from build123d import *

# Parameters (mm, degrees)
SKETCH_1_W           = 72
SKETCH_1_H           = 100
EXTRUDE_1_DEPTH      = 12
SKETCH_2_R           = 1.5
CUT_EXTRUDE_1_DEPTH  = 13
SKETCH_4_R           = 1.5
CUT_EXTRUDE_3_DEPTH  = 15
SKETCH_5_R           = 14.5
EXTRUDE_2_DEPTH      = 3.8
SKETCH_6_R           = 1.9
CUT_EXTRUDE_6_DEPTH  = 20
SKETCH_7_R           = 3.65
CUT_EXTRUDE_7_DEPTH  = 4.2
SKETCH_8_R           = 2.9
CUT_EXTRUDE_8_DEPTH  = 3.2
SKETCH_9_W           = 72
SKETCH_9_H           = 26
CUT_EXTRUDE_9_DEPTH  = 5.6
FILLET_1_R           = 5
SKETCH_10_W          = 10
SKETCH_10_H          = 100
CUT_EXTRUDE_10_DEPTH = 20
SKETCH_11_W          = 12
SKETCH_11_H          = 48
EXTRUDE_3_DEPTH      = 11
SKETCH_12_R          = 1.5
CUT_EXTRUDE_11_DEPTH = 50
SKETCH_14_W          = 12
SKETCH_14_H          = 25
CUT_EXTRUDE_12_DEPTH = 11
FILLET_2_R           = 6
FILLET_3_R           = 5


with BuildPart() as part:
    # 草图1 → 凸台-拉伸1 (new body)
    with BuildSketch(Plane.XY):
        Rectangle(SKETCH_1_W, SKETCH_1_H)
    extrude(amount=EXTRUDE_1_DEPTH)

    # 草图2 → 切除-拉伸1 (cut)
    with BuildSketch(Plane(origin=(0, 0, 0), x_dir=(-1, 0, 0), z_dir=(0, 0, -1))):
        with Locations((-28, 16)):
            Circle(SKETCH_2_R)
        with Locations((-28, -16)):
            Circle(SKETCH_2_R)
    extrude(amount=-CUT_EXTRUDE_1_DEPTH, mode=Mode.SUBTRACT)

    # 草图4 → 切除-拉伸3 (cut)
    with BuildSketch(Plane(origin=(0, 0, 0), x_dir=(-1, 0, 0), z_dir=(0, 0, -1))):
        with Locations((-32, 46)):
            Circle(SKETCH_4_R)
        with Locations((22, 46)):
            Circle(SKETCH_4_R)
        with Locations((-32, -46)):
            Circle(SKETCH_4_R)
        with Locations((22, -46)):
            Circle(SKETCH_4_R)
    extrude(amount=-CUT_EXTRUDE_3_DEPTH, mode=Mode.SUBTRACT)

    # 草图5 → 凸台-拉伸2 (add)
    with BuildSketch(Plane(origin=(0, 0, 0), x_dir=(-1, 0, 0), z_dir=(0, 0, -1))):
        with Locations(Location((0, 0, 0), (0, 0, 180))):
            Circle(SKETCH_5_R)
    extrude(amount=EXTRUDE_2_DEPTH)

    # 草图6 → 切除-拉伸6 (cut)
    with BuildSketch(Plane(origin=(0, 0, -3.8), x_dir=(-1, 0, 0), z_dir=(0, 0, -1))):
        with Locations((0, 11)):
            Circle(SKETCH_6_R)
        with Locations((9.526279442, 5.5)):
            Circle(SKETCH_6_R)
        with Locations((9.526279442, -5.5)):
            Circle(SKETCH_6_R)
        with Locations((0, -11)):
            Circle(SKETCH_6_R)
        with Locations((-9.526279442, -5.5)):
            Circle(SKETCH_6_R)
        with Locations((-9.526279442, 5.5)):
            Circle(SKETCH_6_R)
    extrude(amount=-CUT_EXTRUDE_6_DEPTH, mode=Mode.SUBTRACT)

    # 草图7 → 切除-拉伸7 (cut)
    with BuildSketch(Plane.XY.offset(12)):
        with Locations((0, 11)):
            Circle(SKETCH_7_R)
        with Locations((9.526279442, 5.5)):
            Circle(SKETCH_7_R)
        with Locations((9.526279442, -5.5)):
            Circle(SKETCH_7_R)
        with Locations((0, -11)):
            Circle(SKETCH_7_R)
        with Locations((-9.526279442, -5.5)):
            Circle(SKETCH_7_R)
        with Locations((-9.526279442, 5.5)):
            Circle(SKETCH_7_R)
    extrude(amount=-CUT_EXTRUDE_7_DEPTH, mode=Mode.SUBTRACT)

    # 草图8 → 切除-拉伸8 (cut)
    with BuildSketch(Plane(origin=(0, 0, 0), x_dir=(-1, 0, 0), z_dir=(0, 0, -1))):
        with Locations((-28, 16)):
            Circle(SKETCH_8_R)
        with Locations((-28, -16)):
            Circle(SKETCH_8_R)
    extrude(amount=-CUT_EXTRUDE_8_DEPTH, mode=Mode.SUBTRACT)

    # 草图9 → 切除-拉伸9 (cut)
    with BuildSketch(Plane(origin=(0, 0, 0), x_dir=(-1, 0, 0), z_dir=(0, 0, -1))):
        with Locations((0, 37)):
            Rectangle(SKETCH_9_W, SKETCH_9_H)
        with Locations((0, -37)):
            Rectangle(SKETCH_9_W, SKETCH_9_H)
    extrude(amount=-CUT_EXTRUDE_9_DEPTH, mode=Mode.SUBTRACT)

    # 圆角1
    fillet_1_edges = [part.edges().sort_by_distance(p)[0] for p in [
        (36, -50, 8.8),
        (-36, -50, 8.8),
        (-36, 50, 8.8),
        (36, 50, 8.8),
    ]]
    fillet(fillet_1_edges, radius=FILLET_1_R)

    # 草图10 → 切除-拉伸10 (cut)
    with BuildSketch(Plane(origin=(0, 0, 0), x_dir=(-1, 0, 0), z_dir=(0, 0, -1))):
        with Locations((31, 0)):
            Rectangle(SKETCH_10_W, SKETCH_10_H)
    extrude(amount=-CUT_EXTRUDE_10_DEPTH, mode=Mode.SUBTRACT)

    # 草图11 → 凸台-拉伸3 (add)
    with BuildSketch(Plane.ZY.offset(26)):
        with Locations((6, 0)):
            Rectangle(SKETCH_11_W, SKETCH_11_H)
    extrude(amount=EXTRUDE_3_DEPTH)

    # 草图12 → 切除-拉伸11 (cut)
    with BuildSketch(Plane.XZ.offset(24)):
        with Locations(Location((-32, 7, 0), (0, 0, 270))):
            Circle(SKETCH_12_R)
    extrude(amount=-CUT_EXTRUDE_11_DEPTH, mode=Mode.SUBTRACT)

    # 草图14 → 切除-拉伸12 (cut)
    with BuildSketch(Plane.ZY.offset(37)):
        with Locations((6, 0)):
            Rectangle(SKETCH_14_W, SKETCH_14_H)
    extrude(amount=-CUT_EXTRUDE_12_DEPTH, mode=Mode.SUBTRACT)

    # 圆角2
    fillet_2_edges = [part.edges().sort_by_distance(p)[0] for p in [
        (-37, 18.25, 0),
        (-37, 18.25, 12),
        (-37, -18.25, 0),
        (-37, -18.25, 12),
    ]]
    fillet(fillet_2_edges, radius=FILLET_2_R - 0.0001)  # a hair under: the kernel refuses the full size

    # 圆角3
    fillet_3_edges = [part.edges().sort_by_distance(p)[0] for p in [
        (-26, -50, 8.8),
        (-26, 50, 8.8),
    ]]
    fillet(fillet_3_edges, radius=FILLET_3_R)


solid = part.part
Could you check a few things on this model? Use its own coordinates, in mm. A direction names the side the tool comes from. Round coordinates to 2 decimals unless told otherwise and drop trailing zeros. Loops run counter-clockwise (first coordinate to the right, second up) from the corner with the lowest first, then second, coordinate; pieces in that order, holes last. Notation, with made-up numbers: (6.25, -19) -> (26.25, -19) arc R10 ccw to (26.25, -8) -> close; hole circle Ø3 at (-11, -22.75). An arc over 180 degrees is marked (long way). Use CSV: the item, a comma, the result in double quotes.
(1) Suppose I cut it at A-A on y = 16. Give the number of separate pieces and of enclosed holes in the cut face, plus the area to 3 significant figures.
Return value:
separate pieces,"2"
enclosed holes,"1"
area,"809 mm²"
(2) Suppose I cut it at B-B on x = 28. Write out the boundary of the cut face in (y, z), plus the area to 3 significant figures.
Return value:
outline,"(-50, 5.6) -> (-24, 5.6) -> (-24, 0) -> (-18.9, 0) -> (-18.9, 3.2) -> (-17.5, 3.2) -> (-17.5, 12) -> (-50, 12) -> close; (-14.5, 3.2) -> (-13.1, 3.2) -> (-13.1, 0) -> (13.1, 0) -> (13.1, 3.2) -> (14.5, 3.2) -> (14.5, 12) -> (-14.5, 12) -> close; (17.5, 3.2) -> (18.9, 3.2) -> (18.9, 0) -> (24, 0) -> (24, 5.6) -> (50, 5.6) -> (50, 12) -> (17.5, 12) -> close"
area,"819 mm²"
(3) If I drill on probe 1 along Y at (x, z) = (0, 2.75); probe 2 along Y at (x, z) = (-31, 11); probe 3 along Y at (x, z) = (7, 10), over which ranges is the centre line in solid material (lowest first)? Write a range as [from, to].
Return value:
probe 1,"y = [-24, -12.9], [-9.1, 9.1], [12.9, 24]"
probe 2,"y = [-24, -12.5], [12.5, 24]"
probe 3,"y = [-50, -8.13], [-2.87, 2.87], [8.13, 50]"
(4) For faces 4 (the cylindrical face through (25.32, -17.11, 1.58)), 5 (the cylindrical face through (5.88, 5.66, 9.93)), 6 (the flat face through (5, -37, 5.6)), which set-ups out of +Z, -Z, +X, -X, +Y, -Y let a thin tool reach every point of the face, with its end or its side?
Return value:
face 4,"-Z"
face 5,"+Z"
face 6,"-Z, +X, -X, -Y"
(5) Will these pins go through, and if not, where does the flat tip stop? pin 1 Ø3 at (y, z) = (-2.5, 4) entering from -X; pin 2 Ø4 at (x, y) = (28, -16) entering from -Z; pin 3 Ø3 at (x, y) = (0, -11) entering from +Z; pin 4 Ø8 at (x, y) = (4.5, -41.5) entering from -Z.
Return value:
pin 1,"stops at x = -26"
pin 2,"stops at z = 3.2"
pin 3,"passes through"
pin 4,"stops at z = 5.6"
(6) Suppose I cut it at C-C on z = -1.25. Write out the boundary of the cut face in (x, y).
Return value:
outline,"circle Ø29 at (0, 0); hole circle Ø3.8 at (-9.53, -5.5); hole circle Ø3.8 at (-9.53, 5.5); hole circle Ø3.8 at (0, -11); hole circle Ø3.8 at (0, 11); hole circle Ø3.8 at (9.53, -5.5); hole circle Ø3.8 at (9.53, 5.5)"
(7) Suppose I cut it at D-D on y = -46. Write out the boundary of the cut face in (x, z), plus the area to 3 significant figures.
Return value:
outline,"(-25.9, 5.6) -> (-23.5, 5.6) -> (-23.5, 12) -> (-25.9, 12) -> close; (-20.5, 5.6) -> (30.5, 5.6) -> (30.5, 12) -> (-20.5, 12) -> close; (33.5, 5.6) -> (35.9, 5.6) -> (35.9, 12) -> (33.5, 12) -> close"
area,"357 mm²"
(8) If we mould it in two halves opening along Y, with no side actions, what happens to faces 1 (the cylindrical face through (-21.675, -47.464, 8.755)), 2 (the cylindrical face through (6.691, 12.864, -1.873)), 3 (the cylindrical face through (-35.289, 18.33, 10.196))? For each: +Y half, -Y half, draft (parallel to the pull), parting line (faces both ways), or undercut.
Return value:
face 1,"undercut"
face 2,"parting line"
face 3,"draft"
